Model file for the job. Use its own axes, mm. Round coordinates to 2 decimals unless told otherwise and drop trailing zeros. Loops run counter-clockwise (first coordinate to the right, second up) from the corner with the lowest first, then second, coordinate; pieces in that order, holes last. Notation, with made-up numbers: M 71.25,30 L 112.25,30 A15 cw 112.25,54 Z; hole C 81.5,49.5 d2. An arc over 180 degrees is marked long. Use a Markdown table: item, result. Add a question column.
Q1. Cut at C-C (y = -11.5). Give the cut face in (x, z), plus the area to 3 significant figures.
Q2. Cut at A-A (y = 9.5). Give the cut face in (x, z), plus the area to 3 significant figures.
Q3. Probe line 1 (X direction, y = 16, z = 7); line 2 (Y direction, x = -46, z = 8.75); line 3 (Y direction, x = -77.5, z = 13). List the from-to ranges inside material, lowest first. Write a range as from..to.
Q4. Cut at B-B (z = 12). Give the cut face in (x, y).
Q5. Cut at D-D (y = -31.5). Give the cut face in (x, z), plus the area to 3 significant figures.
Q6. Pin check, flat tips, straight feed: pin 1 (4 mm diameter, centred on y = -26.5, z = 13.5, fed in from -X); pin 2 (6 mm diameter, centred on y = 15.5, z = 3.5, fed in from -X); pin 3 (8 mm diameter, centred on y = -14, z = 6, fed in from -X). Stop position of each tip, or through.
from build123d import *

# Parameters (mm, degrees)
F1_DEPTH = 25.4


with BuildPart() as f1:
    # F0 (on Top) → F1 (new body)
    with BuildSketch(Plane.XY):
        with BuildLine():
            Line((-63.5961517692, -37.6021821231), (-63.5961517692, -37.8618910909))
            Line((-63.5961517692, -37.8618910909), (63.5961517692, -37.8618910909))
            Line((63.5961517692, -37.8618910909), (63.5961517692, 37.8618910909))
            Line((63.5961517692, 37.8618910909), (-63.5961517692, 37.8618910909))
            Line((-63.5961517692, 37.8618910909), (-63.5961517692, 37.6021821231))
            ThreePointArc((-63.5961517692, 37.6021821231), (-37.0073938025, 26.5887579667), (-25.993969646, 0))
            ThreePointArc((-25.993969646, 0), (-37.0073938025, -26.5887579667), (-63.5961517692, -37.6021821231))
        make_face()
        with BuildLine():
            ThreePointArc((-63.5961517692, 37.6021821231), (-101.1983338923, 0), (-63.5961517692, -37.6021821231))
            Line((-63.5961517692, -37.6021821231), (-63.5961517692, -19.1149251528))
            ThreePointArc((-63.5961517692, -19.1149251528), (-82.711076922, 0), (-63.5961517692, 19.1149251528))
            Line((-63.5961517692, 19.1149251528), (-63.5961517692, 37.6021821231))
        make_face()
        with BuildLine():
            Line((-63.5961517692, -19.1149251528), (-63.5961517692, -37.6021821231))
            ThreePointArc((-63.5961517692, -37.6021821231), (-37.0073938025, -26.5887579667), (-25.993969646, 0))
            ThreePointArc((-25.993969646, 0), (-37.0073938025, 26.5887579667), (-63.5961517692, 37.6021821231))
            Line((-63.5961517692, 37.6021821231), (-63.5961517692, 19.1149251528))
            ThreePointArc((-63.5961517692, 19.1149251528), (-50.0798585717, 13.5162931974), (-44.4812266163, 0))
            ThreePointArc((-44.4812266163, 0), (-50.0798585717, -13.5162931974), (-63.5961517692, -19.1149251528))
        make_face()
    extrude(amount=F1_DEPTH)


solid = f1.part
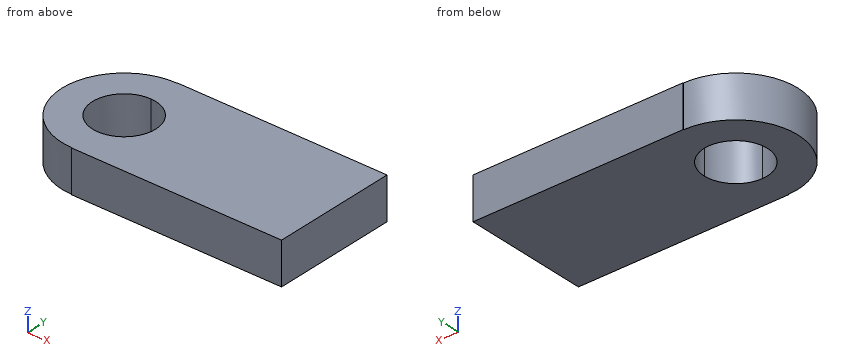
Checked values:
| question | item | result |
|---|---|---|
| 1 | outline | M -99.4,0 L -78.86,0 L -78.86,25.4 L -99.4,25.4 Z; M -48.33,0 L 63.6,0 L 63.6,25.4 L -48.33,25.4 Z |
| 1 | area | 3,360 mm^2 |
| 2 | outline | M -99.98,0 L -80.18,0 L -80.18,25.4 L -99.98,25.4 Z; M -47.01,0 L 63.6,0 L 63.6,25.4 L -47.01,25.4 Z |
| 2 | area | 3,310 mm^2 |
| 3 | line 1 | x = -97.62..-74.05, -53.14..63.6 |
| 3 | line 2 | y = -37.86..-7.47, 7.47..37.86 |
| 3 | line 3 | y = -34.94..-13.12, 13.12..34.94 |
| 4 | outline | M -63.6,-37.86 L 63.6,-37.86 L 63.6,37.86 L -63.6,37.86 L -63.6,37.6 A37.6 ccw -63.6,-37.6 Z; hole C -63.6,0 d38.23 |
| 5 | outline | M -84.13,0 L 63.6,0 L 63.6,25.4 L -84.13,25.4 Z |
| 5 | area | 3,750 mm^2 |
| 6 | pin 1 | stops at x = -92.12 |
| 6 | pin 2 | stops at x = -99.06 |
| 6 | pin 3 | stops at x = -99.84 |
